Verification items for the finished model (mm, model axes). A direction names the side the tool comes from. Give positions to 0.01 mm unless a question says otherwise; leave off trailing zeros. Order: outer loops, then holes, each group sorted by start corner. A loop starts at its lowest first (then second) coordinate and runs counter-clockwise, first axis right, second up. Notation, with made-up numbers: (24, 87.5) -> (28, 87.5) arc R10 cw to (28, 101.5) -> close; hole circle Ø2 at (-2, -13). An arc over 180 degrees is marked (long way). One line per question, with ' | ' between items. Start each with the question number.
Q1. Access from +Z, -Z, +X, -X, +Y, -Y to the whole of each face (thin tool, end or side, straight path). Record for faces 1 (the flat face through (13.72, 27.48, 3.75)), 2 (the flat face through (17, 27, 4)), 3 (the flat face through (22, 15, 5)).
Q2. Material ranges on probe 1 along X at (y, z) = (14.5, 1.95); probe 2 along X at (y, z) = (30.5, 3.75); probe 3 along Y at (x, z) = (30, 3.25), recorded low to high. Write a range as [from, to].
Q3. Mould release check, pull along X, two halves, no side actions. Record for faces 4 (the flat face through (28.2, 21.9, 4.7)), 5 (the flat face through (22, 2, 2)): released by +X, released by -X, zero draft, split by the parting line, or undercut.
Q4. Section check B-B on z = 2.35. Record the cut outline in (x, y).
Q5. Go/stop test with flat-tipped pins: pin 1 (1 mm diameter, centred on x = 36, z = 2, fed in from -Y); pin 2 (2.5 mm diameter, centred on x = 23, z = 2.5, fed in from -Y); pin 3 (3 mm diameter, centred on x = 16.5, z = 5, fed in from -Y). Record where each tip stops, or that it passes through.
Q6. Section check D-D on z = 4.6. Record the cut outline in (x, y), plus the area to 3 significant figures.
Autodesk Inventor part; units mm, degrees
ref_plane "Work Plane4" through (27.5, 27.5, 4) normal (0.7071, -0.7071, 0) x (0, 0, 1)
ref_plane "Work Plane5" through (26.0858, 15.0858, 4) normal (-0.7071, -0.7071, 0) x (0, 0, 1)
ref_plane "YZ Plane" through (0, 0, 0) normal (1, 0, 0) x (0, 1, 0)
sketch "Sketch1" plane through (0, 0, 0) normal (0, 0, 1) x (1, 0, 0)
  line L0 (0, 0) -> (44, 0)
  line L1 (44, 0) -> (44, 44)
  line L2 (44, 44) -> (0, 44)
  line L3 (0, 44) -> (0, 0)
  dimension "d0" = 44
  dimension "d1" = 44
extrude "Extrusion1" add sketch "Sketch1" along normal blind 4
chamfer "Chamfer1" distance 4 angle 45 4 edges at (22, 44, 4) (44, 22, 4) (22, 0, 4) (0, 22, 4)
sketch "Sketch2" plane through (0, 0, 4) normal (0, 0, 1) x (1, 0, 0)
  line L0 (40, 4) -> (4, 4)
  line L1 (40, 40) -> (40, 4)
  line L2 (4, 40) -> (40, 40)
  line L3 (4, 4) -> (4, 40)
  line L4 (40, 4) -> (4, 4)
  line L5 (40, 40) -> (40, 4)
  line L6 (4, 4) -> (40, 40)
  line L7 (4, 40) -> (40, 40)
  line L8 (40, 4) -> (4, 40)
  line L9 (22, 16.5) -> (16.5, 16.5)
  line L10 (16.5, 16.5) -> (16.5, 27.5)
  line L11 (16.5, 27.5) -> (27.5, 27.5)
  line L12 (27.5, 27.5) -> (27.5, 16.5)
  line L13 (27.5, 16.5) -> (22, 16.5)
  line L14 (27.5, 27.5) -> (27.5, 25.5)
  arc A0 (18.5, 27.5) -> (16.5, 25.5) centre (18.5, 25.5) ccw
  line L15 (18.5, 25.5) -> (18.5, 18.5)
  line L16 (18.5, 18.5) -> (25.5, 18.5)
  line L17 (25.5, 18.5) -> (25.5, 25.5)
  arc A1 (16.5, 18.5) -> (18.5, 16.5) centre (18.5, 18.5) ccw
  arc A2 (25.5, 16.5) -> (27.5, 18.5) centre (25.5, 18.5) ccw
  arc A3 (27.5, 25.5) -> (25.5, 27.5) centre (25.5, 25.5) ccw
  line L18 (27.5, 18.5) -> (25.5, 16.5)
  line L19 (18.5, 16.5) -> (16.5, 18.5)
  line L20 (16.5, 25.5) -> (18.5, 27.5)
  line L21 (25.5, 27.5) -> (27.5, 25.5)
  point P0 (0, 0)
  dimension "d86" = 2
extrude "Extrusion2" cut sketch "Sketch2" against normal blind 3 contours L18 L8 L17 L6 L21 L12 | L13 L9 L19 L6 L16 L8 L18 | L10 L20 L8 L15 L6 L19 | L21 L6 L8 L20 L11 | L16 L6 L8 | L8 L6 L17 | L15 L8 L6
ref_plane "Work Plane3" through (27.5, 16.5, 4) normal (-0.7071, -0.7071, 0) x (0, 0, 1)
ref_plane "Work Plane4" through (27.5, 27.5, 4) normal (0.7071, -0.7071, 0) x (0, 0, 1)
ref_plane "Work Plane5" through (26.0858, 15.0858, 4) normal (-0.7071, -0.7071, 0) x (0, 0, 1)
sketch "Sketch13" plane through (27.5, 27.5, 4) normal (0.7071, -0.7071, 0) x (0, 0, 1)
  line L0 (-4.8, 9.7782) -> (0.8, 9.7782)
  line L1 (-3, 9.1924) -> (-3, 14.1421)
  line L2 (-3, 9.7782) -> (-3, 11.0282)
  line L3 (-3, 11.0282) -> (-0.5, 11.0282)
  line L4 (-0.5, 11.0282) -> (-0.5, 8.5282)
  line L5 (-0.5, 8.5282) -> (-3, 8.5282)
  line L6 (-3, 8.5282) -> (-3, 9.7782)
  point P0 (-4, 38.8909)
  point P1 (-3, 9.1924)
  dimension "d88" = 1.25
  dimension "d89" = 2.5
  dimension "d90" = 2.5
sketch "Sketch14" plane through (26.0858, 15.0858, 4) normal (-0.7071, -0.7071, 0) x (0, 0, 1)
  line L0 (-3, 7.7782) -> (-1.75, 7.7782)
  line L1 (-1.75, 7.7782) -> (-1.75, 17.7782)
  line L2 (-1.75, 17.7782) -> (0, 19.5282)
  line L3 (-1.75, 17.7782) -> (0.7249, 17.7782) construction
  line L4 (-1.75, 7.7782) -> (-1.75, -2.2218)
  line L5 (-1.75, -2.2218) -> (0, -3.9718)
  line L6 (0, 19.5282) -> (2.0141, 21.5422)
  line L7 (0, -3.9718) -> (2.0141, -5.9859)
  point P0 (-4, 7.7782)
  dimension "d91" = 1.25
  dimension "d92" = 10
  dimension "d93" = 45
  dimension "d94" = 10
sweep "Sweep3" cut profiles "Sketch13" path "Sketch14" path curves L7 L5 L4 L1 L2 L6
mirror "Mirror2" about plane through (27.5, 16.5, 4) normal (-0.7071, -0.7071, 0) of "Sweep3"
sketch "Sketch15" plane through (0, 0, 4) normal (0, 0, 1) x (1, 0, 0)
  line L0 (17.2396, 31.3566) -> (15.4718, 29.5888)
  line L1 (15.4718, 29.5888) -> (12.9718, 32.0888)
  line L2 (12.9718, 32.0888) -> (14.7396, 33.8566)
  line L3 (14.7396, 33.8566) -> (17.2396, 31.3566)
  line L4 (31.3566, 17.2396) -> (33.8566, 14.7396)
  line L5 (33.8566, 14.7396) -> (32.0888, 12.9718)
  line L6 (32.0888, 12.9718) -> (29.5888, 15.4718)
  line L7 (29.5888, 15.4718) -> (31.3566, 17.2396)
  line L8 (14.4112, 28.5282) -> (12.6434, 26.7604)
  line L9 (12.6434, 26.7604) -> (10.1434, 29.2604)
  line L10 (10.1434, 29.2604) -> (11.9112, 31.0282)
  line L11 (11.9112, 31.0282) -> (14.4112, 28.5282)
  line L12 (29.2604, 10.1434) -> (26.7604, 12.6434)
  line L13 (26.7604, 12.6434) -> (28.5282, 14.4112)
  line L14 (28.5282, 14.4112) -> (31.0282, 11.9112)
  line L15 (31.0282, 11.9112) -> (29.2604, 10.1434)
  line L16 (18.5, 16.5) -> (16.5, 18.5)
  line L17 (16.5, 18.5) -> (16.5, 25.5)
  line L18 (16.5, 25.5) -> (18.5, 27.5)
  line L19 (18.5, 27.5) -> (25.5, 27.5)
  line L20 (25.5, 27.5) -> (27.5, 25.5)
  line L21 (27.5, 25.5) -> (27.5, 18.5)
  line L22 (27.5, 18.5) -> (25.5, 16.5)
  line L23 (25.5, 16.5) -> (18.5, 16.5)
  line L24 (40, 4) -> (4, 4)
  line L25 (40, 40) -> (40, 4)
  line L26 (4, 40) -> (40, 40)
  line L27 (4, 4) -> (4, 40)
  line L28 (16.5, 18.5) -> (16.5, 22.9038)
  line L29 (15, 22.9038) -> (15, 29)
  line L30 (15, 29) -> (29, 29)
  line L31 (29, 29) -> (29, 15)
  line L32 (29, 15) -> (15, 15)
  line L33 (15, 15) -> (15, 29)
  line L34 (16.5, 18.5) -> (16.5, 16.5)
  line L35 (16.5, 16.5) -> (18.5, 16.5)
  line L36 (25.5, 16.5) -> (22.9038, 16.5)
  line L37 (25.5, 16.5) -> (27.5, 16.5)
  line L38 (27.5, 16.5) -> (27.5, 18.5)
  line L39 (27.5, 25.5) -> (27.5, 27.5)
  line L40 (25.5, 27.5) -> (27.5, 25.5)
  line L41 (27.5, 27.5) -> (25.5, 27.5)
  line L42 (18.5, 27.5) -> (16.5, 27.5)
  line L43 (16.5, 27.5) -> (16.5, 25.5)
  point P0 (0, 0)
  dimension "d97" = 1.5
extrude "Extrusion7" add sketch "Sketch15" along normal blind 1.5 contours L29 L30 L31 L32 L33
chamfer "Chamfer6" distance 1.5 angle 45 4 edges at (22, 16.5, 5.5) (16.5, 22, 5.5) (27.5, 22, 5.5) (22, 27.5, 5.5)
properties part number "clear-square-reed"
Filled in:
1) face 1: none | face 2: +Z | face 3: +Z, +X, -X, -Y
2) probe 1: [1.95, 24.9], [28.44, 30.56], [30.72, 42.05] | probe 2: [3.75, 11.74], [12.44, 14.56], [16.74, 40.25] | probe 3: [3.25, 11.94], [12.94, 15.06], [18.6, 40.75]
3) face 4: undercut | face 5: zero draft
4) outline: (2.35, 2.35) -> (41.65, 2.35) -> (41.65, 41.65) -> (2.35, 41.65) -> close; hole (11.31, 28.09) -> (16.5, 22.9) -> (16.5, 18.5) -> (18.5, 16.5) -> (22.9, 16.5) -> (28.09, 11.31) -> (29.86, 13.08) -> (25.97, 16.97) -> (27.03, 18.03) -> (30.92, 14.14) -> (32.69, 15.91) -> (27.5, 21.1) -> (27.5, 25.5) -> (25.5, 27.5) -> (21.1, 27.5) -> (15.91, 32.69) -> (14.14, 30.92) -> (18.03, 27.03) -> (16.97, 25.97) -> (13.08, 29.86) -> close
5) pin 1: y = 1.5 | pin 2: y = 1.25 | pin 3: y = 3.5
6) outline: (15, 15) -> (29, 15) -> (29, 29) -> (15, 29) -> close; hole (15.9, 15.9) -> (28.1, 15.9) -> (28.1, 28.1) -> (15.9, 28.1) -> close | area: 47.2 mm²
